Could you check a few things on this drawing? It's one solid part, dimensions in mm from its lowest x, y, z. Round coordinates to 2 decimals unless told otherwise and drop trailing zeros. Write each loop counter-clockwise with the first axis right and the second up, starting at its lowest first coordinate (ties: lowest second). Pieces come first, ordered by that corner, then holes. Notation, with made-up numbers: M 65,-35.75 L 110,-35.75 A33 ccw 110,-2.75 Z; hole C 57.5,56 d3. An arc over 180 degrees is marked long. One line per item, written item: value. Start each with the question number.
(1) I want a section at D-D on x = 155. Please give me the cut outline in (y, z).
(2) I want a section at B-B on x = 29. Please give me the cut outline in (y, z), and give its area (3 significant figures).
(3) If I drill on L1, parallel to X at y = 60, z = 3.7 (3 decimals); L2, parallel to X at y = 168.5, z = 4.35; L3, parallel to X at y = 10, z = 4.6, over which ranges is the centre line in solid material (lowest first)?
(4) I want a section at C-C on z = 3.85. Count the separate pieces of the cut face and the enclosed holes in it, and give its area (3 significant figures).
(5) I'm going to push flat-ended pins straight in: pin 1 Ø4 at (x, y) = (9, 29) entering from +Z; pin 2 Ø3 at (x, z) = (106, 1.5) entering from +Y; pin 3 Ø2 at (x, z) = (101, 0.5) entering from +Y; pin 4 Ø3 at (y, z) = (157.5, 0.5) entering from +X. Where does each tip first touch, or does it pass through?
(6) I want a section at A-A on y = 169. Please give me the cut outline in (x, z), and give its area (3 significant figures).
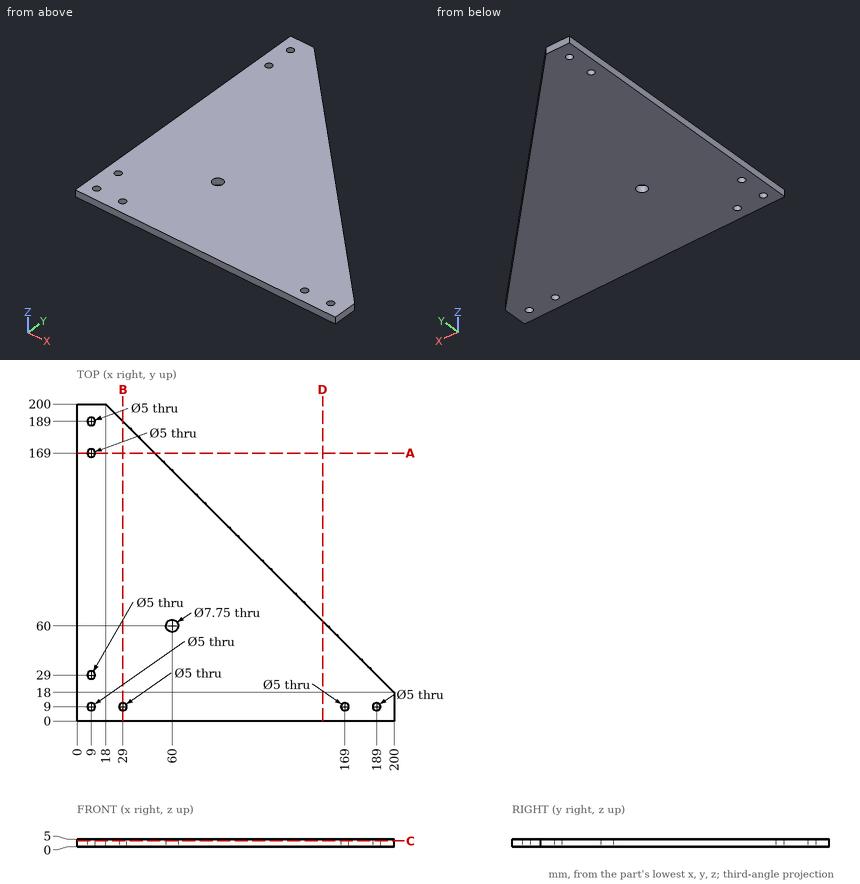
Found:
1. outline: M 0,0 L 63,0 L 63,5 L 0,5 Z
2. outline: M 0,0 L 6.5,0 L 6.5,5 L 0,5 Z; M 11.5,0 L 189,0 L 189,5 L 11.5,5 Z
2. area: 920 mm²
3. L1: x = 0 to 56.125, 63.875 to 158
3. L2: x = 0 to 6.55, 11.45 to 49.5
3. L3: x = 0 to 6.71, 11.29 to 26.71, 31.29 to 166.71, 171.29 to 186.71, 191.29 to 200
4. separate pieces: 1
4. enclosed holes: 8
4. area: 23,300 mm²
5. pin 1: passes through
5. pin 2: stops at y = 113.5
5. pin 3: stops at y = 118
5. pin 4: stops at x = 62
6. outline: M 0,0 L 6.5,0 L 6.5,5 L 0,5 Z; M 11.5,0 L 49,0 L 49,5 L 11.5,5 Z
6. area: 220 mm²
